Can you work these out from the drawing? Everything is in mm from the part's minimum corner. Give positions to 0.01 mm unless a question says otherwise; leave off trailing zeros. Write each loop counter-clockwise with the first axis right and the second up, starting at its lowest first coordinate (ties: lowest second). Pieces come first, ordered by that corner, then holes. Notation, with made-up numbers: (-30, 48.25) - (25, 48.25) arc R23 ccw to (25, 78.25) - close; hole circle Ø2 at (87, 74). An arc over 180 degrees is marked (long way). Return JSON: item names as keys, results as strings. Group by question number.
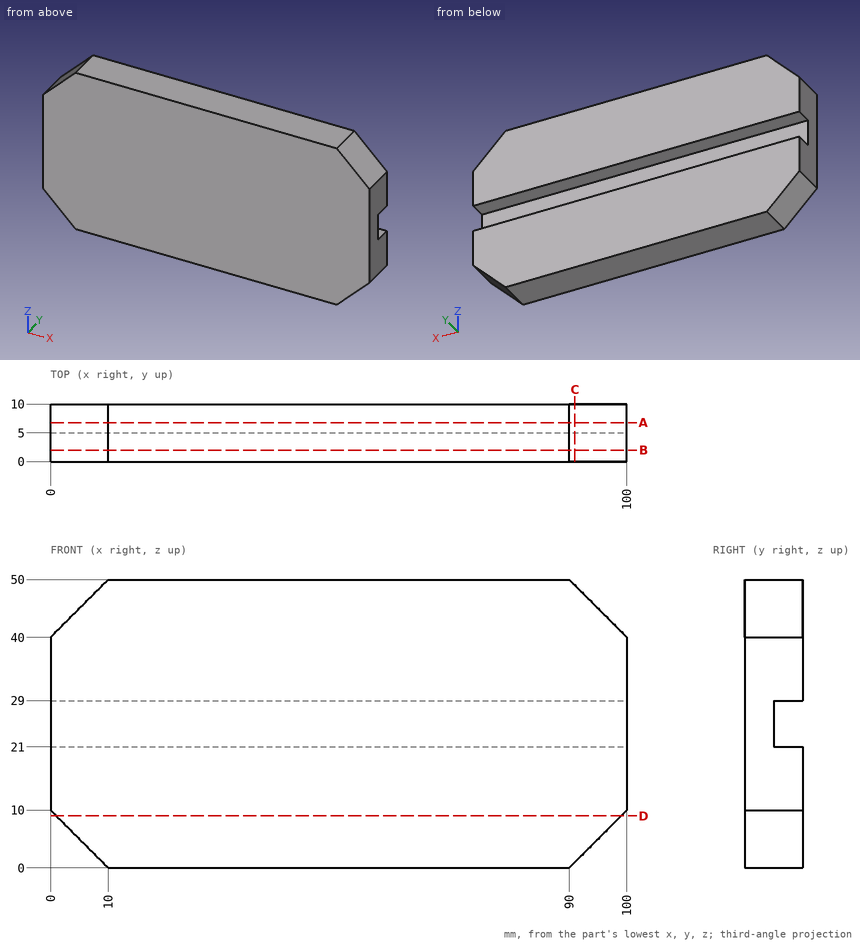
1) Imagine slicing it at B-B, the plane y = 2. Write out the boundary of the cut face in (x, z), and give its area (3 significant figures).
2) Imagine slicing it at C-C, the plane x = 91. Write out the boundary of the cut face in (y, z), and give its area (3 significant figures).
3) Will these pins go through, and if not, where does the flat tip stop? pin 1 Ø2.5 at (x, z) = (28.5, 24) entering from +Y; pin 2 Ø4 at (y, z) = (8.5, 5.5) entering from +X.
4) Imagine slicing it at D-D, the plane z = 9. Write out the boundary of the cut face in (x, y).
5) I need wall thicknesses on line 1 along Z through (x, y) = (50, 9.25); line 2 along Y through (x, z) = (38, 27); line 3 along Z through (x, y) = (9.5, 5.75). Which ranges of each line are inside material? Lowest first, please.
6) Imagine slicing it at A-A, the plane y = 6.75. Write out the boundary of the cut face in (x, z).
Resolved:
{
 "1": {"outline": "(0, 10) - (10, 0) - (90, 0) - (100, 10) - (100, 40) - (90, 50) - (10, 50) - (0, 40) - close", "area": "4,800 mm^2"},
 "2": {"outline": "(0, 1) - (10, 1) - (10, 21) - (5, 21) - (5, 29) - (10, 29) - (10, 49) - (0, 49) - close", "area": "440 mm^2"},
 "3": {"pin 1": "y = 5", "pin 2": "x = 97.5"},
 "4": {"outline": "(1, 0) - (99, 0) - (99, 10) - (1, 10) - close"},
 "5": {"line 1": "0 to 21, 29 to 50", "line 2": "0 to 5", "line 3": "0.5 to 21, 29 to 49.5"},
 "6": {"outline": "(0, 10) - (10, 0) - (90, 0) - (100, 10) - (100, 21) - (0, 21) - close; (0, 29) - (100, 29) - (100, 40) - (90, 50) - (10, 50) - (0, 40) - close"}
}
